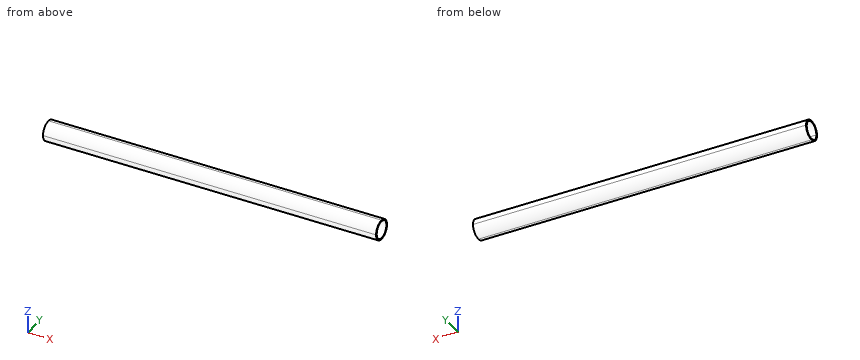
```python
from build123d import *

# Parameters (mm, degrees)
F1_DEPTH = 25
F2_R     = 24.99999
F4_D     = 44
F4_DEPTH = 403.0937720853
F6_D     = 44


# Not quite as in the source:
# - a fillet or chamfer is up to 0.001 mm smaller than in the source, because OpenCascade refuses the exact size


with BuildPart() as f1:
    # F0 (on Top) → F1 (new body, symmetric)
    with BuildSketch(Plane.XY):
        Polygon((446.9072279147, 0), (0, 0), (-403.0927720853, 0), (-403.0927720853, -25), (446.9072279147, -25), align=None)
        Polygon((-403.0927720853, 0), (0, 0), (446.9072279147, 0), (446.9072279147, 25), (-403.0927720853, 25), align=None)
    extrude(amount=F1_DEPTH, both=True)

    # F2 (radius 25 in the source; OpenCascade refuses exactly that, so slightly less here)
    f2_edges = [f1.edges().sort_by_distance(p)[0] for p in [
        (21.907228, -25, -25),
        (21.907228, 25, -25),
        (21.907228, 25, 25),
        (21.907228, -25, 25),
    ]]
    fillet(f2_edges, radius=F2_R)

    # F4 (through all, one way)
    with BuildSketch(Plane.YZ):
        with Locations((0, 0)):
            Circle(F4_D / 2)
    extrude(amount=-F4_DEPTH, mode=Mode.SUBTRACT)

    # F6 (through all)
    with Locations(Plane.YZ.offset(446.9072279147)):
        with Locations((0, 0)):
            Hole(F6_D / 2)


solid = f1.part
```
Geometry: final body of the model. Coordinates: model frame, mm. Coordinates: 2 decimals unless noted, no trailing zeros. Write each loop counter-clockwise with the first axis right and the second up, starting at its lowest first coordinate (ties: lowest second). Pieces come first, ordered by that corner, then holes. Notation, with made-up numbers: M 47.5,51.5 L 92.5,51.5 A18 ccw 92.5,65.5 Z; hole C 84,-12.75 d5. An arc over 180 degrees is marked long. Answer as CSV lines item,"result". Start each with the question number.
Q1. Line query: line 1 (Z direction, x = -51, y = 13); line 2 (Z direction, x = -233, y = -4); line 3 (Y direction, x = -213.5, z = 3.5). Output: solid intervals per line, ascending. Write a range as from..to.
Q2. Cut plane B-B on y = -9. Return the cut outline in (x, z), then the cut area to 3 significant figures.
Q3. Pin query (flat end, axial travel): P1, Ø6, axis at x = -169, y = 19.5, coming from the +Z side; P2, Ø10, axis at x = 347, z = 2, coming from the -Y side; P3, Ø1, axis at x = 5.5, y = -19.5, coming from the -Z side; P4, Ø1.5, axis at x = -133.5, z = 12, coming from the -Y side. Return the tip coordinate at first contact, or that it passes through.
Q4. Cut plane A-A on z = -11.5. Return the cut outline in (x, y) (3 decimals).
Findings below:
1,line 1,"z = -21.35..-17.75, 17.75..21.35"
1,line 2,"z = -24.68..-21.63, 21.63..24.68"
1,line 3,"y = -24.75..-21.72, 21.72..24.75"
2,outline,"M -403.09,-23.32 L 446.91,-23.32 L 446.91,-20.07 L -403.09,-20.07 Z; M -403.09,20.07 L 446.91,20.07 L 446.91,23.32 L -403.09,23.32 Z"
2,area,"5,520 mm2"
3,P1,"stops at z = 18.78"
3,P2,"stops at y = -25"
3,P3,"stops at z = -16.25"
3,P4,"stops at y = -22.33"
4,outline,"M -403.093,-22.198 L 446.907,-22.198 L 446.907,-18.755 L -403.093,-18.755 Z; M -403.093,18.755 L 446.907,18.755 L 446.907,22.198 L -403.093,22.198 Z"
